Autodesk Inventor part; units mm, degrees
ref_plane "YZ Plane" through (0, 0, 0) normal (1, 0, 0) x (0, 1, 0)
ref_plane "XZ Plane" through (0, 0, 0) normal (0, 1, 0) x (-1, 0, 0)
ref_plane "XY Plane" through (0, 0, 0) normal (0, 0, 1) x (1, 0, 0)
sketch "Sketch1" plane through (0, 0, 0) normal (1, 0, 0) x (0, 1, 0)
  line L0 (0, 0) -> (12.7, 0)
  line L1 (12.7, 0) -> (12.7, -901.7)
  line L2 (12.7, -901.7) -> (0, -901.7)
  line L3 (0, -901.7) -> (0, -850.9)
  line L4 (0, -850.9) -> (-12.7, -850.9)
  line L5 (-12.7, -850.9) -> (-12.7, -50.8)
  line L6 (-12.7, -50.8) -> (0, -50.8)
  line L7 (0, -50.8) -> (0, 0)
  dimension "d3" = 12.7
  dimension "d4" = 901.7
  dimension "d5" = 12.7
  dimension "d6" = 50.8
  dimension "d7" = 12.7
  dimension "d8" = 800.1
extrude "Extrusion1" add sketch "Sketch1" along normal mid plane 25.4
properties part number "door top" material "Wood (Cherry)"
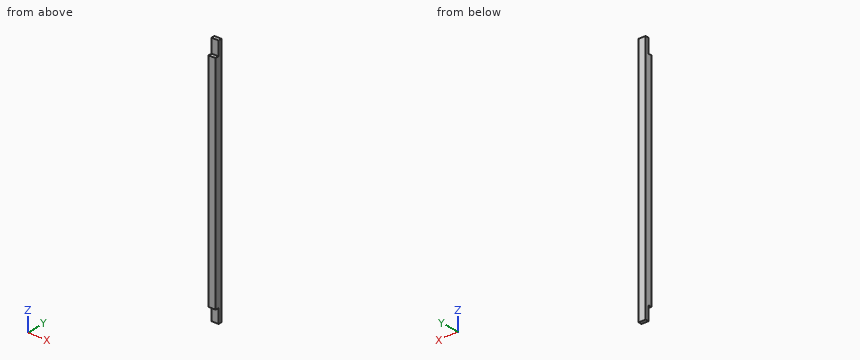
Source: CAD feature listing. Evaluate the final solid. Frame: model axes, mm. Round coordinates to 2 decimals unless told otherwise and drop trailing zeros. Order: outer loops, then holes, each group sorted by start corner. A loop starts at its lowest first (then second) coordinate and runs counter-clockwise, first axis right, second up. Notation, with made-up numbers: (-17, 14) - (38, 14) arc R27 cw to (38, 38) - close; hole circle Ø9 at (9.25, 14). An arc over 180 degrees is marked (long way). Use a Markdown table: item, result. Add a question column.
1. Line query: probe 1 along Z at (x, y) = (11, -7.25). Output: solid intervals per line, ascending.
2. First-contact query: pin 1 (6.5 mm diameter, centred on x = 1, y = -6.5, fed in from +Z); pin 2 (8 mm diameter, centred on x = 9, y = -1.5, fed in from -Z); pin 3 (12.5 mm diameter, centred on x = 6, z = -21.5, fed in from -Y); pin 4 (4 mm diameter, centred on x = 0.5, y = -7, fed in from -Z). Flat tips, straight axial feed; report the tip coordinate or a pass-through.
3. Section query A-A (x = -1.25). Return the cut outline in (y, z).
4. Section query B-B (y = -4.75). Return the cut outline in (x, z), then the cut area to 3 significant figures.
Derived:
| question | item | result |
|---|---|---|
| 1 | probe 1 | -850.9 to -50.8 |
| 2 | pin 1 | z = -50.8 |
| 2 | pin 2 | z = -901.7 |
| 2 | pin 3 | y = 0 |
| 2 | pin 4 | z = -850.9 |
| 3 | outline | (-12.7, -850.9) - (0, -850.9) - (0, -901.7) - (12.7, -901.7) - (12.7, 0) - (0, 0) - (0, -50.8) - (-12.7, -50.8) - close |
| 4 | outline | (-12.7, -850.9) - (12.7, -850.9) - (12.7, -50.8) - (-12.7, -50.8) - close |
| 4 | area | 20,300 mm2 |
